Read the model definition and answer for the solid it produces. Units are mm, in the model's axes. Face numbers are marked on the shaded views. A direction names the side the tool comes from. Coordinates: 2 decimals unless noted, no trailing zeros. Write each loop counter-clockwise with the first axis right and the second up, starting at its lowest first coordinate (ties: lowest second). Pieces come first, ordered by that corner, then holes. Notation, with made-up numbers: (43, -4) -> (77, -4) arc R24 ccw to (77, 23) -> close; hole circle Ø4 at (67, -9). An arc over 180 degrees is marked (long way). Return JSON: item names as keys, results as strings.
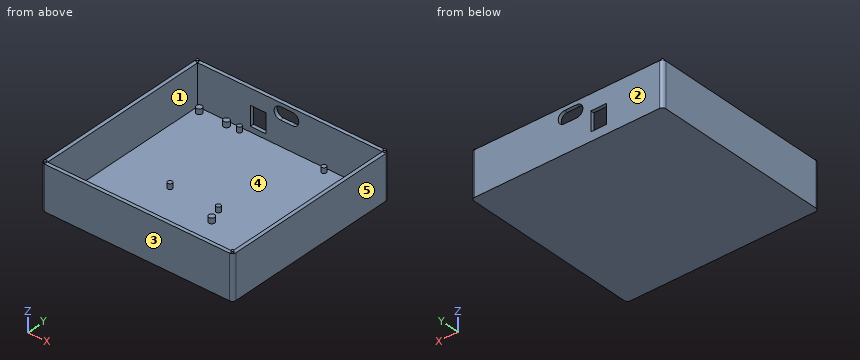
from build123d import *

# Parameters (mm, degrees)
SKETCH_W        = 105
SKETCH_H        = 100
PAD_DEPTH       = 25
PAD001_DEPTH    = 2
SKETCH003_W     = 9
SKETCH003_H     = 11
POCKET_DEPTH    = 5
POCKET001_DEPTH = 2
SKETCH007_R     = 0.7
PAD006_DEPTH    = 1
PAD007_DEPTH    = 2
SKETCH005_R     = 1.3
SKETCH005_R_2   = 1.65
PAD008_DEPTH    = 3


with BuildPart() as part:
    # Sketch → Pad (new body)
    with BuildSketch(Plane.XY):
        with BuildLine():
            Line((-54.5, 50), (-54.5, -50))
            ThreePointArc((-54.5, -50), (-53.914214, -51.414214), (-52.5, -52))
            Line((-52.5, -52), (52.5, -52))
            ThreePointArc((52.5, -52), (53.914214, -51.414214), (54.5, -50))
            Line((54.5, -50), (54.5, 50))
            ThreePointArc((54.5, 50), (53.914214, 51.414214), (52.5, 52))
            Line((52.5, 52), (-52.5, 52))
            ThreePointArc((-52.5, 52), (-53.914214, 51.414214), (-54.5, 50))
        make_face()
        Rectangle(SKETCH_W, SKETCH_H, mode=Mode.SUBTRACT)
    extrude(amount=PAD_DEPTH)

    # Sketch001 → Pad001 (join)
    with BuildSketch(Plane.XY):
        with BuildLine():
            Line((-54.5, 47), (-54.5, -47))
            ThreePointArc((-54.5, -47), (-53.035534, -50.535534), (-49.5, -52))
            Line((-49.5, -52), (49.5, -52))
            ThreePointArc((49.5, -52), (53.035534, -50.535534), (54.5, -47))
            Line((54.5, -47), (54.5, 47))
            ThreePointArc((54.5, 47), (53.035534, 50.535534), (49.5, 52))
            Line((49.5, 52), (-49.5, 52))
            ThreePointArc((-49.5, 52), (-53.035534, 50.535534), (-54.5, 47))
        make_face()
    extrude(amount=PAD001_DEPTH)

    # Sketch003 (on Face13 of Pad001) → Pocket (cut)
    with BuildSketch(Plane(origin=(0, 52, 0), x_dir=(-1, 0, 0), z_dir=(0, 1, 0))):
        with Locations((18.000214, 10.5)):
            Rectangle(SKETCH003_W, SKETCH003_H)
    extrude(amount=-POCKET_DEPTH, mode=Mode.SUBTRACT)

    # Sketch004 (on Face8 of Pocket) → Pocket001 (cut)
    with BuildSketch(Plane(origin=(0, 52, 0), x_dir=(-1, 0, 0), z_dir=(0, 1, 0))):
        with BuildLine():
            ThreePointArc((5.5, 15.9), (9, 19.4), (5.5, 22.9))
            Line((5.5, 22.9), (-1.5, 22.9))
            ThreePointArc((-1.5, 22.9), (-5, 19.4), (-1.5, 15.9))
            Line((5.5, 15.9), (-1.5, 15.9))
        make_face()
    extrude(amount=-POCKET001_DEPTH, mode=Mode.SUBTRACT)

    # Sketch007 → Pad006 (join)
    with BuildSketch(Plane.XY.offset(25)):
        with Locations((53.200001, 50.700001)):
            Circle(SKETCH007_R)
        with Locations((-53.200001, 50.700001)):
            Circle(SKETCH007_R)
        with Locations((-53.200001, -50.700001)):
            Circle(SKETCH007_R)
        with Locations((53.200001, -50.700001)):
            Circle(SKETCH007_R)
    extrude(amount=PAD006_DEPTH)

    # Sketch001 → Pad007 (join)
    with BuildSketch(Plane.XY):
        with BuildLine():
            Line((-54.5, 47), (-54.5, -47))
            ThreePointArc((-54.5, -47), (-53.035534, -50.535534), (-49.5, -52))
            Line((-49.5, -52), (49.5, -52))
            ThreePointArc((49.5, -52), (53.035534, -50.535534), (54.5, -47))
            Line((54.5, -47), (54.5, 47))
            ThreePointArc((54.5, 47), (53.035534, 50.535534), (49.5, 52))
            Line((49.5, 52), (-49.5, 52))
            ThreePointArc((-49.5, 52), (-53.035534, 50.535534), (-54.5, 47))
        make_face()
    extrude(amount=PAD007_DEPTH)

    # Sketch005 (on Face23 of Pocket001) → Pad008 (join)
    with BuildSketch(Plane.XY.offset(2)):
        with Locations((-26.500001, 47.400001)):
            Circle(SKETCH005_R)
        with Locations((-33.500001, 47.000001)):
            Circle(SKETCH005_R_2)
        with Locations((-49.000001, 47.000001)):
            Circle(SKETCH005_R_2)
        with Locations((-49.000001, -37.999999)):
            Circle(SKETCH005_R_2)
        with Locations((-33.500001, -37.999999)):
            Circle(SKETCH005_R_2)
        with Locations((21.499999, 47.400001)):
            Circle(SKETCH005_R)
        with Locations((-21.200001, -5.099999)):
            Circle(SKETCH005_R)
        with Locations((6.299999, -5.099999)):
            Circle(SKETCH005_R)
        with Locations((9.299999, -13.099999)):
            Circle(SKETCH005_R_2)
        with Locations((35.799999, -13.099999)):
            Circle(SKETCH005_R_2)
        with Locations((9.299999, -33.099999)):
            Circle(SKETCH005_R_2)
        with Locations((35.799999, -33.099999)):
            Circle(SKETCH005_R_2)
    extrude(amount=PAD008_DEPTH)


solid = part.part
1. Consider L1, parallel to Y at x = 33, z = 5.75; L2, parallel to X at y = 17.5, z = 13.5; L3, parallel to Z at x = -11, y = -42.5. Determine where each line is inside the solid, lowest interval first.
Taken from the geometry:
{"L1": "y = -52 to -50, 50 to 52", "L2": "x = -54.5 to -52.5, 52.5 to 54.5", "L3": "z = 0 to 2"}
2. The part is cut by section C-C (y = 32). Determine the outline of the cut face in (x, z).
Taken from the geometry:
{"outline": "(-54.5, 0) -> (54.5, 0) -> (54.5, 25) -> (52.5, 25) -> (52.5, 2) -> (-52.5, 2) -> (-52.5, 25) -> (-54.5, 25) -> close"}
3. The part is cut by section A-A (y = -5.1). Determine the outline of the cut face in (x, z).
Taken from the geometry:
{"outline": "(-54.5, 0) -> (54.5, 0) -> (54.5, 25) -> (52.5, 25) -> (52.5, 2) -> (7.6, 2) -> (7.6, 5) -> (5, 5) -> (5, 2) -> (-19.9, 2) -> (-19.9, 5) -> (-22.5, 5) -> (-22.5, 2) -> (-52.5, 2) -> (-52.5, 25) -> (-54.5, 25) -> close"}
4. The part is cut by section B-B (z = 8). Determine the outline of the cut face in (x, y), then the cut area to 3 significant figures.
Taken from the geometry:
{"outline": "(-54.5, -50) arc R2 ccw to (-52.5, -52) -> (52.5, -52) arc R2 ccw to (54.5, -50) -> (54.5, 50) arc R2 ccw to (52.5, 52) -> (-13.5, 52) -> (-13.5, 50) -> (52.5, 50) -> (52.5, -50) -> (-52.5, -50) -> (-52.5, 50) -> (-22.5, 50) -> (-22.5, 52) -> (-52.5, 52) arc R2 ccw to (-54.5, 50) -> close", "area": "815 mm2"}
5. A tool of negligible diameter and unlimited length cuts with its end or side. For the marked faces 4 and 5, from which of +Z, -Z, +X, -X, +Y, -Y can it reach the whole face along a straight path? Write none if from no direction.
Taken from the geometry:
{"face 4": "+Z", "face 5": "+Z, -Z, +X, +Y, -Y"}
6. Flat-ended cylindrical pins translate along their axes: pin 1 Ø1 at (x, y) = (-48.5, -37) entering from +Z; pin 2 Ø6 at (x, y) = (20, -14.5) entering from +Z; pin 3 Ø0.6 at (x, y) = (-20, 51) entering from +Z. Find the tip coordinate at first contact, or state that the pin passes through.
Taken from the geometry:
{"pin 1": "stops at z = 5", "pin 2": "stops at z = 2", "pin 3": "stops at z = 25"}
7. For a pull along Y with two mould halves and no side action, classify the marked faces 1, 2 and 3 as +Y half, -Y half, draft (parallel to the pull), parting line (faces both ways), or undercut.
Taken from the geometry:
{"face 1": "undercut", "face 2": "+Y half", "face 3": "-Y half"}
